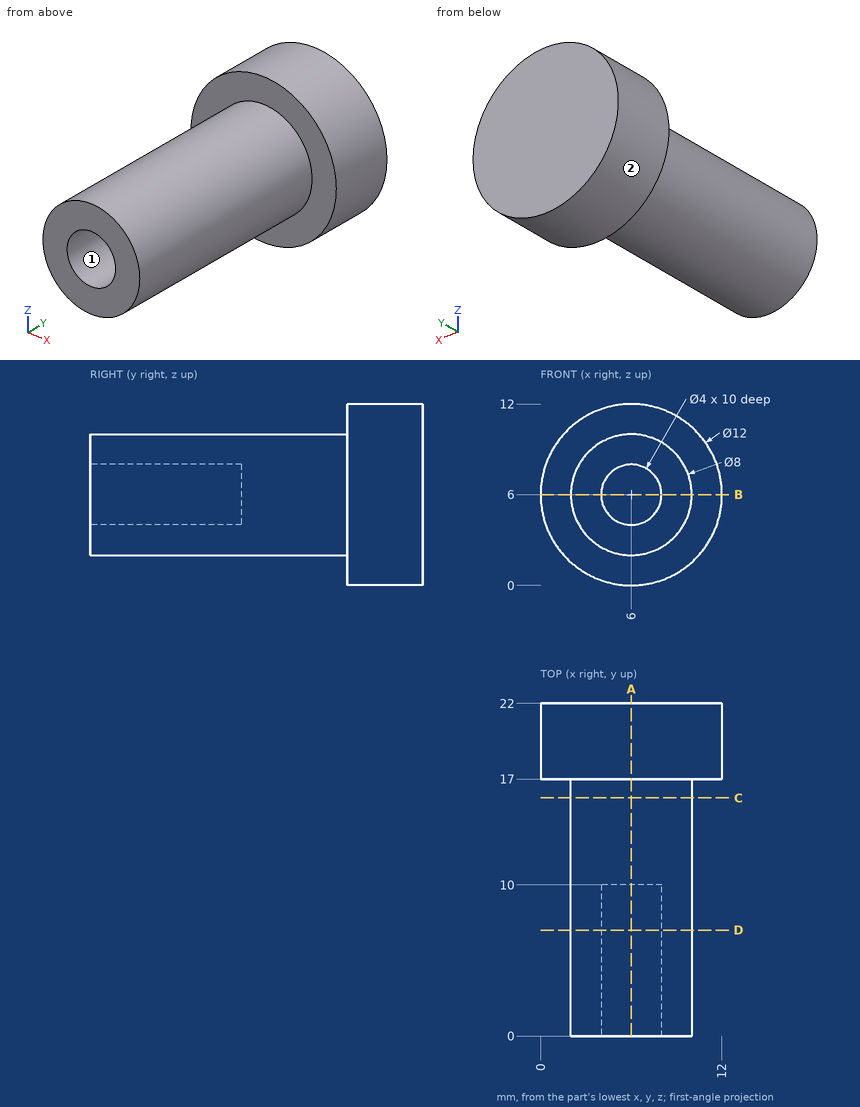
Verification items for this drawing (mm, ordinates from the low corner). A direction names the side the tool comes from. Round coordinates to 2 decimals unless told otherwise and drop trailing zeros. Write each loop counter-clockwise with the first axis right and the second up, starting at its lowest first coordinate (ties: lowest second). Pieces come first, ordered by that corner, then holes. Notation, with made-up numbers: (38, 27) - (77, 27) arc R36 cw to (77, 61) - close; hole circle Ø8 at (41.5, -1). An arc over 180 degrees is marked (long way). Answer as a JSON object with one key per item and string values. Group by question number.
Q1. Section check A-A, the plane x = 6. Enter the section's corners in (y, z), plus the area to 3 significant figures.
Q2. Section check D-D, the plane y = 7. Enter the section's corners in (x, z).
Q3. Go/stop test with flat-tipped pins: pin 1 Ø6 at (y, z) = (11, 1.5) entering from +X; pin 2 Ø5 at (x, y) = (3, 19) entering from -Z; pin 3 Ø3 at (y, z) = (12, 1.5) entering from +X. Record where each tip stops, or that it passes through.
Q4. Section check B-B, the plane z = 6. Enter the section's corners in (x, y), plus the area to 3 significant figures.
Q5. Tool access check on the marked faces 1 and 2. Record the directions out of +Z, -Z, +X, -X, +Y, -Y that give a thin tool (end or side, any length) a straight path to the whole face; none if there is none.
Q6. Thickness scan on line 1 (Z direction, x = 6, y = 3.5); line 2 (Y direction, x = 7, z = 1); line 3 (Y direction, x = 5.5, z = 4.75). Record the ranges inside material, lowest first.
Q7. Section check C-C, the plane y = 15.75. Enter the section's corners in (x, z), plus the area to 3 significant figures.
Found:
{
 "1": {"outline": "(0, 2) - (17, 2) - (17, 0) - (22, 0) - (22, 12) - (17, 12) - (17, 10) - (0, 10) - (0, 8) - (10, 8) - (10, 4) - (0, 4) - close", "area": "156 mm^2"},
 "2": {"outline": "circle Ø8 at (6, 6); hole circle Ø4 at (6, 6)"},
 "3": {"pin 1": "stops at x = 9.71", "pin 2": "stops at z = 0.02", "pin 3": "stops at x = 8.65"},
 "4": {"outline": "(0, 17) - (2, 17) - (2, 0) - (4, 0) - (4, 10) - (8, 10) - (8, 0) - (10, 0) - (10, 17) - (12, 17) - (12, 22) - (0, 22) - close", "area": "156 mm^2"},
 "5": {"face 1": "-Y", "face 2": "+Y, -Y"},
 "6": {"line 1": "z = 2 to 4, 8 to 10", "line 2": "y = 17 to 22", "line 3": "y = 10 to 22"},
 "7": {"outline": "circle Ø8 at (6, 6)", "area": "50.3 mm^2"}
}
